from build123d import *

# Parameters (mm, degrees)
SKETCH1_W           = 65
SKETCH1_H           = 28
SKETCH1_W_2         = 40
SKETCH1_H_2         = 22
BOSS_EXTRUDE1_DEPTH = 1.5
CUT_EXTRUDE1_DEPTH  = 2.5
FILLET2_R           = 1.5


with BuildPart() as part:
    # Sketch1 → Boss-Extrude1 (new body)
    with BuildSketch(Plane(origin=(0, 0, 0), x_dir=(1, 0, 0), z_dir=(0, 1, 0))):
        Rectangle(SKETCH1_W, SKETCH1_H)
        Rectangle(SKETCH1_W_2, SKETCH1_H_2, mode=Mode.SUBTRACT)
    extrude(amount=BOSS_EXTRUDE1_DEPTH)

    # Sketch2 → Cut-Extrude1 (cut, through all)
    with BuildSketch(Plane(origin=(0, 1.5, 0), x_dir=(1, 0, 0), z_dir=(0, 1, 0))):
        with BuildLine():
            Line((-31.1, -12), (-31.1, 12))
            ThreePointArc((-31.1, 12), (-30, 13.1), (-28.9, 12))
            Line((-28.9, 12), (-28.9, -12))
            ThreePointArc((-28.9, -12), (-30, -13.1), (-31.1, -12))
        make_face()
        with BuildLine():
            Line((31.1, -12), (31.1, 12))
            ThreePointArc((31.1, 12), (30, 13.1), (28.9, 12))
            Line((28.9, 12), (28.9, -12))
            ThreePointArc((28.9, -12), (30, -13.1), (31.1, -12))
        make_face()
    extrude(amount=-CUT_EXTRUDE1_DEPTH, mode=Mode.SUBTRACT)

    # Fillet2
    fillet2_edges = [part.edges().sort_by_distance(p)[0] for p in [
        (32.5, 0.75, 14),
        (-32.5, 0.75, 14),
        (-32.5, 0.75, -14),
        (32.5, 0.75, -14),
    ]]
    fillet(fillet2_edges, radius=FILLET2_R)


solid = part.part
For this review, take the finished solid that the model builds, in its own axes (mm). A direction names the side the tool comes from. Give positions to 0.01 mm unless a question says otherwise; leave off trailing zeros. Write each loop counter-clockwise with the first axis right and the second up, starting at its lowest first coordinate (ties: lowest second). Pieces come first, ordered by that corner, then holes. Notation, with made-up numbers: (27.25, 36.25) -> (34.25, 36.25) arc R24 ccw to (34.25, 47.25) -> close; hole circle Ø6 at (62.25, 64). An arc over 180 degrees is marked (long way). Use CSV: the item, a comma, the result in double quotes.
Q1. Take a section at B-B, the plane y = 1.25. Write out the cut boundary in (x, z), then the cut area to 3 significant figures.
Conclusion:
outline,"(-32.5, -12.5) arc R1.5 ccw to (-31, -14) -> (31, -14) arc R1.5 ccw to (32.5, -12.5) -> (32.5, 12.5) arc R1.5 ccw to (31, 14) -> (-31, 14) arc R1.5 ccw to (-32.5, 12.5) -> close; hole (-31.1, -12) arc R1.1 ccw to (-28.9, -12) -> (-28.9, 12) arc R1.1 ccw to (-31.1, 12) -> close; hole (-20, -11) -> (20, -11) -> (20, 11) -> (-20, 11) -> close; hole (28.9, -12) arc R1.1 ccw to (31.1, -12) -> (31.1, 12) arc R1.1 ccw to (28.9, 12) -> close"
area,"825 mm2"
Q2. Tool access review of faces 1 (the face through (32.5, 1, 0)), 2 (the face through (-28.9, 1, 0)): name each direction out of +Z, -Z, +X, -X, +Y, -Y from which nothing blocks a thin tool from reaching the whole face with its end or side.
Conclusion:
face 1,"+Z, -Z, +X, +Y, -Y"
face 2,"+Y, -Y"
Q3. Mouldability with a two-part tool opening along X and no side actions: class faces 3 (the face through (-32.07, 0.76, -13.55)), 4 (the face through (0, 1, 14)), 5 (the face through (20, 1, 0)) as pulls with the +X half, pulls with the -X half, needs draft (parallel to the pull), parting line crosses it, or undercut.
Conclusion:
face 3,"pulls with the -X half"
face 4,"needs draft"
face 5,"undercut"
Q4. Take a section at C-C, the plane x = -30. Write out the cut boundary in (y, z), then the cut area to 3 significant figures.
Conclusion:
outline,"(0, -14) -> (1.5, -14) -> (1.5, -13.1) -> (0, -13.1) -> close; (0, 13.1) -> (1.5, 13.1) -> (1.5, 14) -> (0, 14) -> close"
area,"2.70 mm2"
Q5. Take a section at D-D, the plane x = 16.5. Write out the cut boundary in (y, z), then the cut area to 3 significant figures.
Conclusion:
outline,"(0, -14) -> (1.5, -14) -> (1.5, -11) -> (0, -11) -> close; (0, 11) -> (1.5, 11) -> (1.5, 14) -> (0, 14) -> close"
area,"9.00 mm2"
Q6. To check wall thickness, follow probe 1 along X at (y, z) = (1.1, -3); probe 2 along X at (y, z) = (0.5, 12); probe 3 along Z at (x, y) = (-2, 0.25). State the ranges of each line that lie inside material, in increasing order. Write a range as [from, to].
Conclusion:
probe 1,"[-32.5, -31.1], [-28.9, -20], [20, 28.9], [31.1, 32.5]"
probe 2,"[-32.5, -31.1], [-28.9, 28.9], [31.1, 32.5]"
probe 3,"[-14, -11], [11, 14]"
Q7. Take a section at A-A, the plane z = -7.25. Write out the cut boundary in (x, y).
Conclusion:
outline,"(-32.5, 0) -> (-31.1, 0) -> (-31.1, 1.5) -> (-32.5, 1.5) -> close; (-28.9, 0) -> (-20, 0) -> (-20, 1.5) -> (-28.9, 1.5) -> close; (20, 0) -> (28.9, 0) -> (28.9, 1.5) -> (20, 1.5) -> close; (31.1, 0) -> (32.5, 0) -> (32.5, 1.5) -> (31.1, 1.5) -> close"
